Source: three-view drawing plus pictorial views. Frame: mm from the lowest corner of the part. Give positions to 0.01 mm unless a question says otherwise; leave off trailing zeros. Loops run counter-clockwise (first coordinate to the right, second up) from the corner with the lowest first, then second, coordinate; pieces in that order, holes last. Notation, with made-up numbers: (41, 25) - (67, 25) arc R13 ccw to (67, 43) - close; hole circle Ø11 at (22, 16). An arc over 180 degrees is marked (long way). Write each question's results on one line, items separated by ' | '. Start each with the question number.
(1) Contact query for flat-ended pins moving along their axis: pin 1 (19 mm diameter, centred on y = 70, z = 450, fed in from -X); pin 2 (1.5 mm diameter, centred on x = 1010, z = 656, fed in from +Y); pin 3 (12 mm diameter, centred on y = 67, z = 456, fed in from +X). Output: stop coordinate, or through.
(2) Cut plane B-B on z = 373.5. Return the cut outline in (x, y), then the cut area to 3 significant figures.
(3) Material intervals for line 1 along Z through (x, y) = (858, 93); line 2 along Y through (x, z) = (1016.5, 176); line 3 along X through (y, z) = (86, 376.5), sorted ascending. Write a range as [from, to].
(4) Cut plane A-A on y = 74. Return the cut outline in (x, z).
(5) Pull-direction query (X, two-part tool) for the marked faces 1 and 2; classes: pulls with the +X half, pulls with the -X half, needs draft (parallel to the pull), parting line crosses it, or undercut.
(6) Cut plane C-C on x = 694. Return the cut outline in (y, z), then the cut area to 3 significant figures.
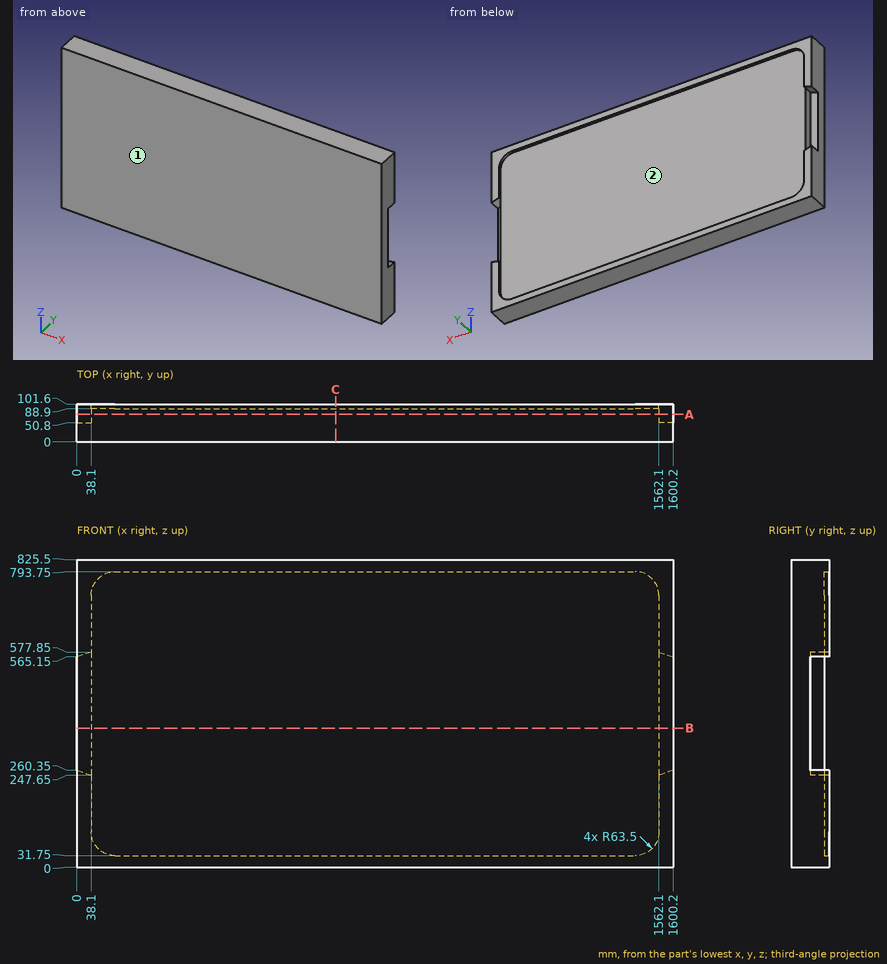
Ans:
1) pin 1: x = 38.1 | pin 2: y = 88.9 | pin 3: x = 1562.1
2) outline: (0, 0) - (1600.2, 0) - (1600.2, 50.8) - (1562.1, 50.8) - (1562.1, 88.9) - (38.1, 88.9) - (38.1, 50.8) - (0, 50.8) - close | area: 139,000 mm^2
3) line 1: [0, 31.75], [793.75, 825.5] | line 2: [0, 88.9] | line 3: [38.1, 1562.1]
4) outline: (0, 0) - (1600.2, 0) - (1600.2, 260.35) - (1562.1, 247.65) - (1562.1, 577.85) - (1600.2, 565.15) - (1600.2, 825.5) - (0, 825.5) - (0, 565.15) - (38.1, 577.85) - (38.1, 247.65) - (0, 260.35) - close
5) face 1: needs draft | face 2: undercut
6) outline: (0, 0) - (101.6, 0) - (101.6, 31.75) - (88.9, 31.75) - (88.9, 793.75) - (101.6, 793.75) - (101.6, 825.5) - (0, 825.5) - close | area: 74,200 mm^2
